Geometry check sheet. Reference: the model listing, model coordinates, mm. A direction names the side the tool comes from. Coordinates: 2 decimals unless noted, no trailing zeros. Write each loop counter-clockwise with the first axis right and the second up, starting at its lowest first coordinate (ties: lowest second). Pieces come first, ordered by that corner, then holes. Notation, with made-up numbers: M 64.5,23.25 L 78.5,23.25 A25 ccw 78.5,45.25 Z; hole C -4.5,-14 d4. An arc over 180 degrees is marked long. Put each result on its own line as item: value. Start each with the question number.
1) Gauge pin test, flat ends, axial feed: pin 1 (10 mm diameter, centred on x = -10, y = -77, fed in from +Z); pin 2 (5 mm diameter, centred on x = 15, z = 11, fed in from +Y); pin 3 (4 mm diameter, centred on x = -18, z = -23.5, fed in from +Y); pin 4 (16 mm diameter, centred on x = 0, y = 0, fed in from -Z). Record the tip position at first contact, or that the pin passes through.
2) Cross-section at B-B on y = 0. Record the cut outline in (x, z), plus the area to 3 significant figures.
3) Mould release check, pull along Y, two halves, no side actions. Record for faces 4 (the flat face through (1.21, -63.7, 13.55)), 5 (the flat face through (1.15, -69.4, 19.79)), 6 (the flat face through (9, -7, 28.5)): released by +Y, released by -Y, zero draft, split by the parting line, or undercut.
4) Set-up check for faces 1 (the flat face through (18.37, 97.16, 9.4)), 2 (the flat face through (-24.829, -111.207, -29.79)), 3 (the cylindrical face through (21.63, 118, -31.37)): record each of +Z, -Z, +X, -X, +Y, -Y from which the full face is reachable in a straight line by a thin tool's end or side.
5) Cross-section at A-A on x = 0. Count the separate pieces of the cut face and the enclosed holes in it, plus the area to 3 significant figures.
6) Cross-section at C-C on y = 78.5. Record the cut outline in (x, z), plus the area to 3 significant figures.
7) Scan lines: line 1 along Y through (x, z) = (0, 21); line 2 along Z through (x, y) = (8.5, -29); line 3 along Z through (x, y) = (1, 73). Record each from-to range of solid material in increasing order.
from build123d import *

# Parameters (mm, degrees)
SKETCH1_R               = 10
BOSS_EXTRUDE1_DEPTH     = 28.5
BOSS_EXTRUDE2_DEPTH     = 45
SKETCH4_R               = 4.7625
SKETCH4_R_2             = 3.96875
CUT_EXTRUDE1_DEPTH      = 258.595725096
FILLET3_R               = 15
SKETCH10_R              = 4
CUT_EXTRUDE2_DEPTH      = 78.869968284
CUT_EXTRUDE2_DEPTH_BACK = 46.869968284
CUT_EXTRUDE4_DEPTH      = 22.5


with BuildPart() as part:
    # Sketch1 → Boss-Extrude1 (new body)
    with BuildSketch(Plane.XY):
        Polygon((-7.617068705, -126.66669812), (39.062241625, 120.733646626), (7.617068705, 126.66669812), (-39.062241625, -120.733646626), align=None)
        Circle(SKETCH1_R, mode=Mode.SUBTRACT)
    extrude(amount=BOSS_EXTRUDE1_DEPTH)

    # Sketch2 → Boss-Extrude2 (add)
    with BuildSketch(Plane(origin=(0, 0, 0), x_dir=(-1, 0, 0), z_dir=(0, 0, -1))):
        Polygon((-39.062241625, 120.733646626), (-36.837347314, 108.941706781), (-5.392174394, 114.874758275), (-7.617068705, 126.66669812), align=None)
        Polygon((36.837347314, -108.941706781), (5.392174394, -114.874758275), (7.617068705, -126.66669812), (39.062241625, -120.733646626), align=None)
    extrude(amount=BOSS_EXTRUDE2_DEPTH)

    # Sketch4 → Cut-Extrude1 (cut, through all)
    with BuildSketch(Plane(origin=(-1.656161502, 128.416364197, 0), x_dir=(0.982661654, -0.185407859, 0), z_dir=(0.185407859, 0.982661654, 0))):
        with Locations((25.436849572, 26.64759704)):
            Circle(SKETCH4_R)
        with Locations((25.436849572, 39)):
            Circle(SKETCH4_R_2)
    extrude(amount=-CUT_EXTRUDE1_DEPTH, mode=Mode.SUBTRACT)

    # Fillet3
    fillet3_edges = [part.edges().sort_by_distance(p)[0] for p in [
        (21.114760854, 111.908232528, 0),
        (-21.114760854, -111.908232528, 0),
    ]]
    fillet(fillet3_edges, radius=FILLET3_R)

    # Sketch10 → Cut-Extrude2 (cut, two sides)
    with BuildSketch(Plane(origin=(-16.024269994, 1.367603019, 0), x_dir=(0, 0, -1), z_dir=(0.982661654, -0.185407859, 0))) as cut_extrude2_sk:
        with Locations((-17.5, 21.627134551)):
            Circle(SKETCH10_R)
        with Locations((-17.5, -18.372865449)):
            Circle(SKETCH10_R)
        with BuildLine():
            Line((-28.5, 31.627134551), (-11.316666773, 106.545885621))
            ThreePointArc((-11.316666773, 106.545885621), (-1.82302812, 121.628280107), (15, 127.509906002))
            Line((15, 127.509906002), (-44.768549469, 140.171550448))
            Line((-44.768549469, 140.171550448), (-46.912682998, 31.416920937))
            Line((-46.912682998, 31.416920937), (-28.5, 31.627134551))
        make_face()
        with BuildLine():
            Line((-44.768549469, -136.917281346), (15, -124.255636901))
            ThreePointArc((15, -124.255636901), (-1.82302812, -118.374011006), (-11.316666773, -103.29161652))
            Line((-11.316666773, -103.29161652), (-28.5, -28.372865449))
            Line((-28.5, -28.372865449), (-46.912682998, -28.162651835))
            Line((-46.912682998, -28.162651835), (-44.768549469, -136.917281346))
        make_face()
    extrude(amount=CUT_EXTRUDE2_DEPTH, mode=Mode.SUBTRACT)
    extrude(cut_extrude2_sk.sketch, amount=-CUT_EXTRUDE2_DEPTH_BACK, mode=Mode.SUBTRACT)

    # Sketch11 → Cut-Extrude4 (cut)
    with BuildSketch(Plane.XY.offset(28.5)):
        with BuildLine():
            Line((3.541290111, 34.949381459), (9.437260033, 33.836934304))
            ThreePointArc((9.437260033, 33.836934304), (16.92877427, 35.404052106), (21.117955163, 41.809472249))
            Line((21.117955163, 41.809472249), (29.254165873, 84.931389014))
            ThreePointArc((29.254165873, 84.931389014), (27.687048071, 92.422903251), (21.281627928, 96.612084144))
            Line((21.281627928, 96.612084144), (15.385658005, 97.724531299))
            ThreePointArc((15.385658005, 97.724531299), (7.894143769, 96.157413497), (3.704962876, 89.751993354))
            Line((3.704962876, 89.751993354), (-4.431247835, 46.630076588))
            ThreePointArc((-4.431247835, 46.630076588), (-2.864130032, 39.138562352), (3.541290111, 34.949381459))
        make_face()
        with BuildLine():
            Line((-21.281627928, -96.612084144), (-15.385658005, -97.724531299))
            ThreePointArc((-15.385658005, -97.724531299), (-7.894143769, -96.157413497), (-3.704962876, -89.751993354))
            Line((-3.704962876, -89.751993354), (4.431247835, -46.630076588))
            ThreePointArc((4.431247835, -46.630076588), (2.864130032, -39.138562352), (-3.541290111, -34.949381459))
            Line((-3.541290111, -34.949381459), (-9.437260033, -33.836934304))
            ThreePointArc((-9.437260033, -33.836934304), (-16.92877427, -35.404052106), (-21.117955163, -41.809472249))
            Line((-21.117955163, -41.809472249), (-29.254165873, -84.931389014))
            ThreePointArc((-29.254165873, -84.931389014), (-27.687048071, -92.422903251), (-21.281627928, -96.612084144))
        make_face()
    extrude(amount=-CUT_EXTRUDE4_DEPTH, mode=Mode.SUBTRACT)


solid = part.part
Answer key:
1. pin 1: stops at z = 6
1. pin 2: stops at y = 111.35
1. pin 3: stops at y = -112.21
1. pin 4: passes through
2. outline: M -16.28,0 L -10,0 L -10,28.5 L -16.28,28.5 Z; M 10,0 L 16.28,0 L 16.28,28.5 L 10,28.5 Z
2. area: 358 mm²
3. face 4: undercut
3. face 5: released by -Y
3. face 6: zero draft
4. face 1: +Z
4. face 2: -Z, +X, +Y
4. face 3: none
5. separate pieces: 2
5. enclosed holes: 2
5. area: 2,370 mm²
6. outline: M -1.47,0 L 31.09,0 L 31.09,16.37 L 28.04,16.5 L 28.04,6 L 1.58,6 L 1.58,17.62 L -1.47,17.75 Z
6. area: 263 mm²
7. line 1: y = -36.36 to -22.32, -18.38 to -10, 10 to 18.38, 22.32 to 36.36
7. line 2: z = 0 to 28.5
7. line 3: z = 0 to 6
